Build history of the part. All positions in model axes, mm. Face numbers are marked on the shaded views. A direction names the side the tool comes from. Round coordinates to 2 decimals unless told otherwise and drop trailing zeros. Write each loop counter-clockwise with the first axis right and the second up, starting at its lowest first coordinate (ties: lowest second). Pieces come first, ordered by that corner, then holes.
1) Wall check: probe 1 along Y at (x, z) = (73, -5.5); probe 2 along X at (y, z) = (-24.5, -6.5); probe 3 along X at (y, z) = (30.5, 28). Give the ranges that are in metal, low to high.
2) Flat gauge pins, fed straight in: pin 1 (3 mm diameter, centred on y = 21.5, z = 3.5, fed in from +X); pin 2 (9.5 mm diameter, centred on x = 26.5, z = 8.5, fed in from -Y); pin 3 (19 mm diameter, centred on y = 1, z = 13.5, fed in from -X). Where does each tip first touch, or does it go through?
3) Which spindle directions (+Z, -Z, +X, -X, +Y, -Y) get a long thin tool onto all of the face, cutting with end or side? Do the marked faces 4, 5 and 6. Say none if no direction does.
4) Saw through at C-C (x = 76). Write the cut outline in (y, z), plus the area to 3 significant figures.
5) Saw through at B-B (z = 23.5). Write the cut outline in (x, y), plus the area to 3 significant figures.
6) Saw through at D-D (y = 16). Write the cut outline in (x, z).
7) Pull direction X, two halves, no side cores. Call the marked faces 1, 2 and 3: +X half, -X half, draft (parallel to the pull), parting line (faces both ways), or undercut.
8) Saw through at A-A (x = 38). Write the cut outline in (y, z), plus the area to 3 significant figures.
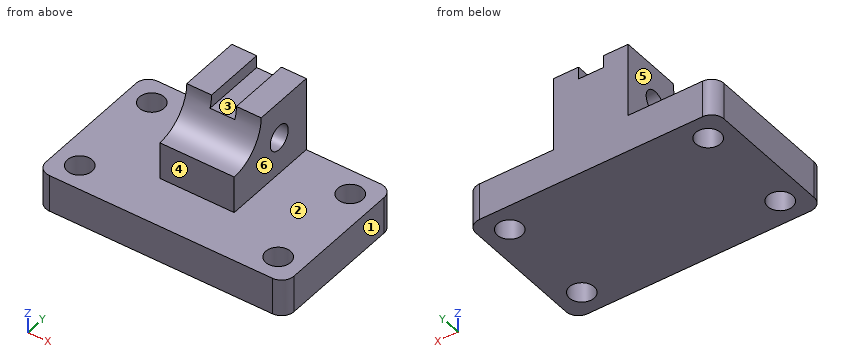
from build123d import *

# Parameters (mm, degrees)
F0_W     = 127
F0_H     = 76.2
F0_R     = 6.35
F1_DEPTH = 19.05
F2_W     = 38.1
F2_H     = 50.8
F3_DEPTH = 38.1
F4_R     = 19.05
F5_DEPTH = 82.551
F6_W     = 12.7
F6_H     = 38.2500794058
F7_DEPTH = 6.35
F8_R     = 6.35
F9_DEPTH = 82.551
F10_R    = 6.35


with BuildPart() as f1:
    # F0 (on Top) → F1 (new body)
    with BuildSketch(Plane.XY):
        with Locations((21.6519124806, 0.1500794058)):
            Rectangle(F0_W, F0_H)
        with Locations((-29.1480875194, -25.2499205942)):
            Circle(F0_R, mode=Mode.SUBTRACT)
        with Locations((72.4519124806, -25.2499205942)):
            Circle(F0_R, mode=Mode.SUBTRACT)
        with Locations((-29.1480875194, 25.5500794058)):
            Circle(F0_R, mode=Mode.SUBTRACT)
        with Locations((72.4519124806, 25.5500794058)):
            Circle(F0_R, mode=Mode.SUBTRACT)
    extrude(amount=-F1_DEPTH)

    # F2 (on face) → F3 (join)
    with BuildSketch(Plane.XY):
        with Locations((21.6519124806, 12.8500794058)):
            Rectangle(F2_W, F2_H)
    extrude(amount=F3_DEPTH)

    # F4 (on face) → F5 (cut, through all)
    with BuildSketch(Plane.YZ.offset(40.7019124806)):
        with Locations((-12.5499205942, 38.1)):
            Circle(F4_R)
    extrude(amount=-F5_DEPTH, mode=Mode.SUBTRACT)

    # F6 (on face) → F7 (cut)
    with BuildSketch(Plane.XY.offset(38.1)):
        with Locations((21.6519124806, 19.1250397029)):
            Rectangle(F6_W, F6_H)
    extrude(amount=-F7_DEPTH, mode=Mode.SUBTRACT)

    # F8 (on face) → F9 (cut, through all)
    with BuildSketch(Plane.YZ.offset(40.7019124806)):
        with Locations((19.2000794058, 19.05)):
            Circle(F8_R)
    extrude(amount=-F9_DEPTH, mode=Mode.SUBTRACT)

    # F10
    f10_edges = [f1.edges().sort_by_distance(p)[0] for p in [
        (-41.848088, -37.949921, -9.525),
        (-41.848088, 38.250079, -9.525),
        (85.151912, -37.949921, -9.525),
        (85.151912, 38.250079, -9.525),
    ]]
    fillet(f10_edges, radius=F10_R)


solid = f1.part
Evaluation:
1. probe 1: y = -37.95 to -31.58, -18.92 to 19.22, 31.88 to 38.25
1. probe 2: x = -41.85 to -35.45, -22.84 to 66.15, 78.76 to 85.15
1. probe 3: x = 2.6 to 40.7
2. pin 1: stops at x = 40.7
2. pin 2: stops at y = -12.55
2. pin 3: stops at x = 2.6
3. face 4: +Z, +X, -X, -Y
3. face 5: +Z, -X, +Y, -Y
3. face 6: +Z, +X, +Y, -Y
4. outline: (-37.95, -19.05) - (-30.52, -19.05) - (-30.52, 0) - (-37.95, 0) - close; (-19.98, -19.05) - (20.28, -19.05) - (20.28, 0) - (-19.98, 0) - close; (30.82, -19.05) - (38.25, -19.05) - (38.25, 0) - (30.82, 0) - close
4. area: 1,050 mm2
5. outline: (2.6, -0.31) - (40.7, -0.31) - (40.7, 14.67) - (2.6, 14.67) - close; (2.6, 23.73) - (40.7, 23.73) - (40.7, 38.25) - (2.6, 38.25) - close
5. area: 1,120 mm2
6. outline: (-41.85, -19.05) - (85.15, -19.05) - (85.15, 0) - (40.7, 0) - (40.7, 13.57) - (2.6, 13.57) - (2.6, 0) - (-41.85, 0) - close; (2.6, 24.53) - (40.7, 24.53) - (40.7, 38.1) - (28, 38.1) - (28, 31.75) - (15.3, 31.75) - (15.3, 38.1) - (2.6, 38.1) - close
7. face 1: +X half
7. face 2: draft
7. face 3: undercut
8. outline: (-37.95, -19.05) - (38.25, -19.05) - (38.25, 38.1) - (6.5, 38.1) arc R19.05 cw to (-12.55, 19.05) - (-12.55, 0) - (-37.95, 0) - close; hole circle Ø12.7 at (19.2, 19.05)
8. area: 2,980 mm2
